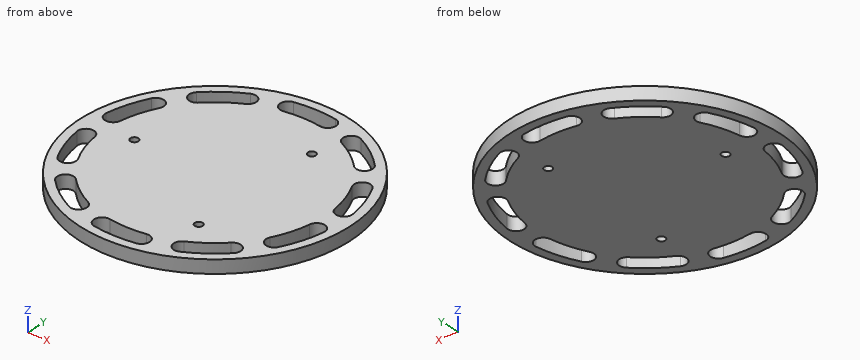
from build123d import *

# Parameters (mm, degrees)
SKETCH015_R        = 51
SKETCH015_R_2      = 1.5
PAD013_DEPTH       = 5
POCKET001_DEPTH    = 5
POLARPATTERN_COUNT = 10


with BuildPart() as part:
    # Sketch015 → Pad013 (new body)
    with BuildSketch(Plane.XY):
        Circle(SKETCH015_R)
        with Locations((15.375, 26.630281)):
            Circle(SKETCH015_R_2, mode=Mode.SUBTRACT)
        with Locations((-30.75, 0)):
            Circle(SKETCH015_R_2, mode=Mode.SUBTRACT)
        with Locations((15.375, -26.630281)):
            Circle(SKETCH015_R_2, mode=Mode.SUBTRACT)
    extrude(amount=-PAD013_DEPTH)

    # Sketch025 → Pocket001 (cut)
    with BuildSketch(Plane.XY):
        with BuildLine():
            ThreePointArc((8.022472, 46.919079), (0, 47.6), (-8.022472, 46.919079))
            ThreePointArc((-8.022472, 46.919079), (-10.555654, 43.340952), (-6.977528, 40.80777))
            ThreePointArc((6.977528, 40.80777), (0, 41.4), (-6.977528, 40.80777))
            ThreePointArc((6.977528, 40.80777), (10.555654, 43.340952), (8.022472, 46.919079))
        make_face()
    pocket001 = extrude(amount=-POCKET001_DEPTH, mode=Mode.SUBTRACT)

    # PolarPattern: Pocket001 ×10 about axis
    polarpattern_axis = Axis((0, 0, 0), (0, 0, 1))
    for i in range(1, POLARPATTERN_COUNT):
        add(pocket001.rotate(polarpattern_axis, i * 360 / POLARPATTERN_COUNT), mode=Mode.SUBTRACT)


solid = part.part
Source: CAD feature listing. Evaluate the final solid. Frame: model axes, mm. Coordinates: 2 decimals unless noted, no trailing zeros. Loops run counter-clockwise (first coordinate to the right, second up) from the corner with the lowest first, then second, coordinate; pieces in that order, holes last. Notation, with made-up numbers: (-17.75, 7) - (-3.75, 7) arc R20 cw to (-3.75, 38) - close; hole circle Ø10 at (42, 29.5). An arc over 180 degrees is marked (long way). One line per item, written item: value. Start each with the question number.
1. Ray query, L1, parallel to X at y = 9.5, z = -0.35; L2, parallel to Y at x = 19.5, z = -0.15; L3, parallel to X at y = -13.5, z = -3.35. Return the intervals inside material, ascending.
2. Section C-C (y = -11.5). Return the cut outline in (x, z), and give its area (3 significant figures).
3. Section D-D (z = -2.95). State how many separate pieces and enclosed holes the cut face has, and give its area (3 significant figures).
4. Contact query for flat-ended pins moving along their axis: P1, Ø1.5, axis at x = -29, z = -3.5, coming from the +Y side; P2, Ø1.5, axis at x = -2.5, z = -1, coming from the -Y side. Output: stop coordinate, or through.
5. Section A-A (x = 0). Return the cut outline in (y, z), and give its area (3 significant figures).
6. Section B-B (y = 0). Return the cut outline in (x, z), and give its area (3 significant figures).
Verdict:
1. L1: x = -50.11 to -46.64, -40.3 to 40.3, 46.64 to 50.11
1. L2: y = -47.12 to -42.99, -36.52 to 36.52, 42.99 to 47.12
1. L3: x = -49.18 to -45.65, -39.14 to 39.14, 45.65 to 49.18
2. outline: (-49.69, -5) - (-46.19, -5) - (-46.19, 0) - (-49.69, 0) - close; (-39.77, -5) - (39.77, -5) - (39.77, 0) - (-39.77, 0) - close; (46.19, -5) - (49.69, -5) - (49.69, 0) - (46.19, 0) - close
2. area: 433 mm2
3. separate pieces: 1
3. enclosed holes: 13
3. area: 6,910 mm2
4. P1: stops at y = 42.46
4. P2: stops at y = -50.97
5. outline: (-51, -5) - (-47.6, -5) - (-47.6, 0) - (-51, 0) - close; (-41.4, -5) - (41.4, -5) - (41.4, 0) - (-41.4, 0) - close; (47.6, -5) - (51, -5) - (51, 0) - (47.6, 0) - close
5. area: 448 mm2
6. outline: (-51, -5) - (-32.25, -5) - (-32.25, 0) - (-51, 0) - close; (-29.25, -5) - (51, -5) - (51, 0) - (-29.25, 0) - close
6. area: 495 mm2
